Can you work these out from the model? Positions are in its coordinate system, mm. A direction names the side the tool comes from. Coordinates: 2 decimals unless noted, no trailing zeros. Order: outer loops, then holes, each group sorted by start corner. A loop starts at its lowest first (then second) coordinate and runs counter-clockwise, first axis right, second up. Notation, with made-up numbers: (11.5, 69) -> (46.5, 69) arc R17 ccw to (46.5, 96) -> close; hole circle Ø5 at (22, -15). An arc over 180 degrees is marked (long way). Answer in a Markdown table with one row per item.
```python
from build123d import *

# Parameters (mm, degrees)
F1_DEPTH     = 2
F3_DEPTH     = 5
F5_DEPTH     = 2
F6_W         = 6.2
F6_H         = 9.1
F7_DEPTH     = 7.001
F8_T1_DEPTH  = 9.1
F8_T3_DEPTH  = 6.2
F8_T9_DEPTH  = 8.771682988
F8_T13_DEPTH = 11.671682988
F8_T20_DEPTH = 11.671682988
F8_T24_DEPTH = 8.771682988
F8_T31_DEPTH = 8.771682988
F8_T36_DEPTH = 11.671682988
F8_T44_DEPTH = 8.771682988
F8_T48_DEPTH = 11.671682988
F8_T55_DEPTH = 8.771682988
F8_T59_DEPTH = 11.671682988
F8_T66_DEPTH = 8.771682988
F8_T70_DEPTH = 11.671682988
F8_T77_DEPTH = 8.771682988
F8_T81_DEPTH = 11.671682988
F8_T88_DEPTH = 11.671682988
F8_T92_DEPTH = 8.771682988
F9_SIZE      = 1.99999


# Not quite as in the source:
# - a fillet or chamfer that OpenCascade refuses, or shapes differently, is made with other operations: its cross-section is extruded or revolved along the edge and cut away or added
# - a fillet or chamfer is up to 0.001 mm smaller than in the source, because OpenCascade refuses the exact size


with BuildPart() as f1:
    # F0 (on Top) → F1 (new body)
    with BuildSketch(Plane.XY):
        Polygon((0, 36), (0, 0), (36, 0), align=None)
    extrude(amount=F1_DEPTH)

    # F2 (on face) → F3 (join)
    with BuildSketch(Plane.XY.offset(2)):
        Polygon((0, 29), (0, 0), (29, 0), align=None)
    extrude(amount=F3_DEPTH)

    # F4 (on face) → F5 (join)
    with BuildSketch(Plane.XY.offset(7)):
        Polygon((29, 0), (0, 29), (0, 26.1715728753), (26.1715728753, 0), align=None)
    extrude(amount=F5_DEPTH)

    # F6 (on face) → F7 (cut, through all)
    with BuildSketch(Plane.XY.offset(7)):
        with Locations((7.1, 9.55)):
            Rectangle(F6_W, F6_H)
    extrude(amount=-F7_DEPTH, mode=Mode.SUBTRACT)

    # F8: chamfer of 1 on 8 edges, made by hand

    # F8_s2 → F8_t1 (cut)
    with BuildSketch(Plane.XZ.offset(-14.1)):
        Polygon((3, 7), (4, 6), (4, 7), align=None)
        Polygon((11.2, 7), (10.2, 6), (10.2, 7), align=None)
        Polygon((11.2, 0), (10.2, 1), (10.2, 0), align=None)
        Polygon((3, 0), (4, 1), (4, 0), align=None)
    extrude(amount=F8_T1_DEPTH, mode=Mode.SUBTRACT)

    # F8_s4 → F8_t3 (cut)
    with BuildSketch(Plane.YZ.offset(4)):
        Polygon((15.1, 7), (14.1, 6), (14.1, 7), align=None)
        Polygon((4, 7), (5, 6), (5, 7), align=None)
        Polygon((15.1, 0), (14.1, 1), (14.1, 0), align=None)
        Polygon((4, 0), (5, 1), (5, 0), align=None)
    extrude(amount=F8_T3_DEPTH, mode=Mode.SUBTRACT)


with BuildPart() as f8_tool7:
    # F8_s8 → F8_t9 (new body)
    with BuildSketch(Plane.YZ.offset(10.2)):
        Polygon((15.1, 7), (14.1, 6), (14.1, 7), align=None)
    extrude(amount=-F8_T9_DEPTH)

    split(bisect_by=Plane.YZ.offset(4), keep=Keep.BOTTOM)


with BuildPart() as f8_tool11:
    # F8_s12 → F8_t13 (new body)
    with BuildSketch(Plane.XZ.offset(-16.671682988)):
        Polygon((3, 7), (4, 6), (4, 7), align=None)
    extrude(amount=F8_T13_DEPTH)

    split(bisect_by=Plane.XZ.offset(-14.1), keep=Keep.BOTTOM)


with BuildPart() as f8_tool7_1:
    add(f8_tool7.part)

    # F8_t15: intersect F8_tool11
    add(f8_tool11.part, mode=Mode.INTERSECT)


with BuildPart() as f1_1:
    add(f1.part)

    # F8_t5: cut F8_tool7
    add(f8_tool7_1.part, mode=Mode.SUBTRACT)


with BuildPart() as f8_tool18:
    # F8_s19 → F8_t20 (new body)
    with BuildSketch(Plane.XZ.offset(-14.1)):
        Polygon((3, 7), (4, 6), (4, 7), align=None)
    extrude(amount=F8_T20_DEPTH)

    split(bisect_by=Plane.XZ.offset(-5), keep=Keep.TOP)


with BuildPart() as f8_tool22:
    # F8_s23 → F8_t24 (new body)
    with BuildSketch(Plane.YZ.offset(1.428317012)):
        Polygon((4, 7), (5, 6), (5, 7), align=None)
    extrude(amount=F8_T24_DEPTH)

    split(bisect_by=Plane.YZ.offset(4), keep=Keep.BOTTOM)


with BuildPart() as f8_tool18_1:
    add(f8_tool18.part)

    # F8_t26: intersect F8_tool22
    add(f8_tool22.part, mode=Mode.INTERSECT)


with BuildPart() as f1_2:
    add(f1_1.part)

    # F8_t16: cut F8_tool18
    add(f8_tool18_1.part, mode=Mode.SUBTRACT)


with BuildPart() as f8_tool29:
    # F8_s30 → F8_t31 (new body)
    with BuildSketch(Plane.YZ.offset(12.771682988)):
        Polygon((15.1, 7), (14.1, 6), (14.1, 7), align=None)
    extrude(amount=-F8_T31_DEPTH)

    split(bisect_by=Plane(origin=(13.0857864376, 13.0857864376, 0), x_dir=(0, 0, 1), z_dir=(-0.7071067812, -0.7071067812, 0)), keep=Keep.TOP)

    split(bisect_by=Plane.YZ.offset(10.2), keep=Keep.TOP)


with BuildPart() as f8_tool34:
    # F8_s35 → F8_t36 (new body)
    with BuildSketch(Plane.XZ.offset(-5)):
        Polygon((11.2, 7), (10.2, 6), (10.2, 7), align=None)
    extrude(amount=-F8_T36_DEPTH)

    split(bisect_by=Plane(origin=(13.0857864376, 13.0857864376, 0), x_dir=(0, 0, 1), z_dir=(-0.7071067812, -0.7071067812, 0)), keep=Keep.TOP)

    split(bisect_by=Plane.XZ.offset(-14.1), keep=Keep.BOTTOM)


with BuildPart() as f8_tool29_1:
    add(f8_tool29.part)

    # F8_t39: intersect F8_tool34
    add(f8_tool34.part, mode=Mode.INTERSECT)


with BuildPart() as f1_3:
    add(f1_2.part)

    # F8_t27: cut F8_tool29
    add(f8_tool29_1.part, mode=Mode.SUBTRACT)


with BuildPart() as f8_tool42:
    # F8_s43 → F8_t44 (new body)
    with BuildSketch(Plane.YZ.offset(4)):
        Polygon((4, 7), (5, 6), (5, 7), align=None)
    extrude(amount=F8_T44_DEPTH)

    split(bisect_by=Plane.YZ.offset(10.2), keep=Keep.TOP)


with BuildPart() as f8_tool46:
    # F8_s47 → F8_t48 (new body)
    with BuildSketch(Plane.XZ.offset(-2.428317012)):
        Polygon((11.2, 7), (10.2, 6), (10.2, 7), align=None)
    extrude(amount=-F8_T48_DEPTH)

    split(bisect_by=Plane.XZ.offset(-5), keep=Keep.TOP)


with BuildPart() as f8_tool42_1:
    add(f8_tool42.part)

    # F8_t50: intersect F8_tool46
    add(f8_tool46.part, mode=Mode.INTERSECT)


with BuildPart() as f1_4:
    add(f1_3.part)

    # F8_t40: cut F8_tool42
    add(f8_tool42_1.part, mode=Mode.SUBTRACT)


with BuildPart() as f8_tool53:
    # F8_s54 → F8_t55 (new body)
    with BuildSketch(Plane.YZ.offset(12.771682988)):
        Polygon((15.1, 0), (14.1, 1), (14.1, 0), align=None)
    extrude(amount=-F8_T55_DEPTH)

    split(bisect_by=Plane.YZ.offset(10.2), keep=Keep.TOP)


with BuildPart() as f8_tool57:
    # F8_s58 → F8_t59 (new body)
    with BuildSketch(Plane.XZ.offset(-5)):
        Polygon((11.2, 0), (10.2, 1), (10.2, 0), align=None)
    extrude(amount=-F8_T59_DEPTH)

    split(bisect_by=Plane.XZ.offset(-14.1), keep=Keep.BOTTOM)


with BuildPart() as f8_tool53_1:
    add(f8_tool53.part)

    # F8_t61: intersect F8_tool57
    add(f8_tool57.part, mode=Mode.INTERSECT)


with BuildPart() as f1_5:
    add(f1_4.part)

    # F8_t51: cut F8_tool53
    add(f8_tool53_1.part, mode=Mode.SUBTRACT)


with BuildPart() as f8_tool64:
    # F8_s65 → F8_t66 (new body)
    with BuildSketch(Plane.YZ.offset(10.2)):
        Polygon((15.1, 0), (14.1, 1), (14.1, 0), align=None)
    extrude(amount=-F8_T66_DEPTH)

    split(bisect_by=Plane.YZ.offset(4), keep=Keep.BOTTOM)


with BuildPart() as f8_tool68:
    # F8_s69 → F8_t70 (new body)
    with BuildSketch(Plane.XZ.offset(-16.671682988)):
        Polygon((3, 0), (4, 1), (4, 0), align=None)
    extrude(amount=F8_T70_DEPTH)

    split(bisect_by=Plane.XZ.offset(-14.1), keep=Keep.BOTTOM)


with BuildPart() as f8_tool64_1:
    add(f8_tool64.part)

    # F8_t72: intersect F8_tool68
    add(f8_tool68.part, mode=Mode.INTERSECT)


with BuildPart() as f1_6:
    add(f1_5.part)

    # F8_t62: cut F8_tool64
    add(f8_tool64_1.part, mode=Mode.SUBTRACT)


with BuildPart() as f8_tool75:
    # F8_s76 → F8_t77 (new body)
    with BuildSketch(Plane.YZ.offset(4)):
        Polygon((4, 0), (5, 1), (5, 0), align=None)
    extrude(amount=F8_T77_DEPTH)

    split(bisect_by=Plane.YZ.offset(10.2), keep=Keep.TOP)


with BuildPart() as f8_tool79:
    # F8_s80 → F8_t81 (new body)
    with BuildSketch(Plane.XZ.offset(-2.428317012)):
        Polygon((11.2, 0), (10.2, 1), (10.2, 0), align=None)
    extrude(amount=-F8_T81_DEPTH)

    split(bisect_by=Plane.XZ.offset(-5), keep=Keep.TOP)


with BuildPart() as f8_tool75_1:
    add(f8_tool75.part)

    # F8_t83: intersect F8_tool79
    add(f8_tool79.part, mode=Mode.INTERSECT)


with BuildPart() as f1_7:
    add(f1_6.part)

    # F8_t73: cut F8_tool75
    add(f8_tool75_1.part, mode=Mode.SUBTRACT)


with BuildPart() as f8_tool86:
    # F8_s87 → F8_t88 (new body)
    with BuildSketch(Plane.XZ.offset(-14.1)):
        Polygon((3, 0), (4, 1), (4, 0), align=None)
    extrude(amount=F8_T88_DEPTH)

    split(bisect_by=Plane.XZ.offset(-5), keep=Keep.TOP)


with BuildPart() as f8_tool90:
    # F8_s91 → F8_t92 (new body)
    with BuildSketch(Plane.YZ.offset(1.428317012)):
        Polygon((4, 0), (5, 1), (5, 0), align=None)
    extrude(amount=F8_T92_DEPTH)

    split(bisect_by=Plane.YZ.offset(4), keep=Keep.BOTTOM)


with BuildPart() as f8_tool86_1:
    add(f8_tool86.part)

    # F8_t94: intersect F8_tool90
    add(f8_tool90.part, mode=Mode.INTERSECT)


with BuildPart() as f1_8:
    add(f1_7.part)

    # F8_t84: cut F8_tool86
    add(f8_tool86_1.part, mode=Mode.SUBTRACT)

    # F9 (size 2 in the source; OpenCascade refuses exactly that, so slightly less here)
    f9_edges = [f1_8.edges().sort_by_distance(p)[0] for p in [
        (18, 18, 0),
    ]]
    chamfer(f9_edges, length=F9_SIZE)


solid = f1_8.part
```
(1) We'd pull the mould along X, two halves only. Please class faces 6 (the flat face through (7.1, 14.6, 6.5)), 7 (the flat face through (13.4, 13.5, 9)), 8 (the flat face through (17.535, 17.031, 0.986)), 9 (the flat face through (0, 14, 3)): +X half, -X half, draft (parallel to the pull), parting line (faces both ways), or undercut.
Response values:
| item | result |
|---|---|
| face 6 | undercut |
| face 7 | draft |
| face 8 | +X half |
| face 9 | -X half |
(2) On a 3-axis mill with a long thin cutter (end or side, diameter ignored), from which of +Z, -Z, +X, -X, +Y, -Y can I reach the whole of each face in a straight line? I mean faces 1 (the flat face through (4, 9, 4)), 2 (the flat face through (12.9, 13.27, 7.95)), 3 (the flat face through (15, 14, 5)), 4 (the flat face through (3.5, 9.6, 6.5)), 5 (the flat face through (10.7, 9.5, 0.5)). Say none if no direction works.
Response values:
| item | result |
|---|---|
| face 1 | +Z, -Z |
| face 2 | +Z, -X, -Y |
| face 3 | +Z, +X, +Y |
| face 4 | +Z |
| face 5 | -Z |
(3) I need wall thicknesses on line 1 (Y direction, x = 20, z = 6.75); line 2 (Z direction, x = 5.5, y = 25); line 3 (Y direction, x = 5, z = 4.75). Which ranges of each line are inside material? Lowest first, please. Write a range as [from, to].
Response values:
| item | result |
|---|---|
| line 1 | [0, 9] |
| line 2 | [0, 2] |
| line 3 | [0, 5], [14.1, 24] |
(4) Will these pins go through, and if not, where does the flat tip stop? pin 1 Ø11 at (x, y) = (12.5, 13) entering from +Z; pin 2 Ø6 at (x, y) = (28.5, 9) entering from -Z; pin 3 Ø2.5 at (x, z) = (6.5, 3.5) entering from +Y; pin 4 Ø1.5 at (y, z) = (10.5, 3) entering from +X.
Response values:
| item | result |
|---|---|
| pin 1 | z = 9 |
| pin 2 | z = 0.06 |
| pin 3 | y = 23.75 |
| pin 4 | x = 19.25 |
(5) Suppose I cut it at A-A (z = 3.75). Please give me the cut outline in (x, y), and give its area (3 significant figures).
Response values:
| item | result |
|---|---|
| outline | (0, 0) -> (29, 0) -> (0, 29) -> close; hole (4, 5) -> (10.2, 5) -> (10.2, 14.1) -> (4, 14.1) -> close |
| area | 364 mm2 |
